Verification items for the finished model (mm, model axes). Face numbers are marked on the shaded views. A direction names the side the tool comes from. Coordinates: 2 decimals unless noted, no trailing zeros. Order: outer loops, then holes, each group sorted by start corner. A loop starts at its lowest first (then second) coordinate and runs counter-clockwise, first axis right, second up. Notation, with made-up numbers: M -37,5 L -11,5 A30 ccw -11,36 Z; hole C -28,-8.5 d7. An arc over 180 degrees is marked long. Write item = value, one per line.
Autodesk Fusion 360 part; units mm, degrees
sketch "Sketch2" plane through (0, 0, 0) normal (1, 0, 0) x (0, 1, 0) in component "Support Batt"
  circle A0 centre (154.2359, 79.3135) radius 4
  line L0 (99.2359, 44.7135) -> (119.2359, 44.7135)
  line L1 (119.2359, 31.7135) -> (119.2359, 44.7135)
  line L2 (99.2359, 31.7135) -> (99.2359, 44.7135)
  line L3 (160.5859, 85.8135) -> (106.4359, 85.8135)
  line L4 (50.5431, 31.7135) -> (52.3447, 31.7135)
  line L5 (52.3447, 31.7135) -> (217.041, 31.7135) construction
  line L6 (96.4359, 75.8135) -> (96.4359, 31.7135)
  line L7 (96.4359, 31.7135) -> (98.9359, 31.7135)
  line L8 (98.9359, 44.7135) -> (119.5359, 44.7135)
  line L9 (119.5359, 44.7135) -> (119.5359, 31.7135)
  line L10 (98.9359, 44.7135) -> (98.9359, 31.7135)
  line L11 (119.5359, 31.7135) -> (122.0359, 31.7135)
  line L12 (154.2359, 83.3135) -> (160.5859, 83.3135) construction
  line L13 (160.5859, 85.8135) -> (160.5859, 70.8135)
  line L14 (158.0859, 70.8135) -> (160.5859, 70.8135)
  line L15 (158.0859, 78.2283) -> (158.0859, 70.8135)
  line L16 (150.3859, 78.2283) -> (150.3859, 70.8135)
  line L17 (150.3859, 70.8135) -> (147.8859, 70.8135)
  line L18 (150.3859, 70.8135) -> (158.0859, 70.8135) construction
  line L19 (154.2359, 79.3135) -> (154.2359, 70.8135) construction
  line L20 (147.8859, 70.8135) -> (147.8859, 71.8135)
  line L21 (137.8859, 81.8135) -> (110.4359, 81.8135)
  line L22 (122.0359, 31.7135) -> (122.0359, 47.7135)
  line L23 (122.0359, 47.7135) -> (110.4359, 47.7135)
  line L24 (100.4359, 57.7135) -> (100.4359, 71.8135)
  arc A1 (110.4359, 81.8135) -> (100.4359, 71.8135) centre (110.4359, 71.8135) ccw
  arc A2 (147.8859, 71.8135) -> (137.8859, 81.8135) centre (137.8859, 71.8135) ccw
  arc A3 (100.4359, 57.7135) -> (110.4359, 47.7135) centre (110.4359, 57.7135) ccw
  arc A4 (158.0859, 78.2283) -> (150.3859, 78.2283) centre (154.2359, 79.3135) ccw
  arc A5 (106.4359, 85.8135) -> (96.4359, 75.8135) centre (106.4359, 75.8135) ccw
  line L25 (114.8859, 81.8135) -> (117.8859, 81.8135)
  line L26 (117.8859, 81.8135) -> (117.8859, 78.8135)
  line L27 (117.8859, 78.8135) -> (114.8859, 78.8135)
  line L28 (114.8859, 78.8135) -> (114.8859, 81.8135)
  line L29 (160.5859, 85.8135) -> (185.5859, 85.8135)
  line L30 (185.5859, 85.8135) -> (185.5859, 82.8135)
  line L31 (185.5859, 82.8135) -> (160.5859, 82.8135)
  line L32 (160.5859, 82.8135) -> (160.5859, 85.8135)
  line L33 (160.5859, 70.8135) -> (185.5859, 82.8135)
  point P0 (96.4359, 85.8135)
  point P1 (100.4359, 81.8135)
  dimension "d2" = 0.3
  dimension "d3" = 0.3
  dimension "d4" = 2.5
  dimension "d5" = 2.5
  dimension "d6" = 2.5
  dimension "d7" = 2.5
  dimension "d8" = 8
  dimension "d9" = 15
  dimension "d10" = 7.7
  dimension "d11" = 2.5
  dimension "d12" = 4
  dimension "d13" = 4
  dimension "d14" = 3
  dimension "d15" = 10
  dimension "d68" = 10
  dimension "d69" = 3
  dimension "d70" = 3
  dimension "d71" = 30
  dimension "d80" = 25
  dimension "d81" = 3
extrude "Extrude1" add sketch "Sketch2" along normal blind 40 contours A0 L0 L3 L6 L7 L8 L9 L10 L11 L13 L14 L15 L16 L17 L20 L21 L22 L23 L24 A1 A2 A3 A4 A5 L25 L32 | L13 L29 L30 L31 L32 | L21 L25 L26 L27 L28 in component "Support Batt"
sketch "Sketch3" plane through (0, 0, 44.7135) normal (0, 0, -1) x (1, 0, 0) in component "Support Batt"
  line L0 (0, -98.9359) -> (0, -119.5359)
  line L1 (0, -119.5359) -> (40, -119.5359)
  line L2 (40, -119.5359) -> (40, -98.9359)
  line L3 (40, -98.9359) -> (0, -98.9359)
  line L4 (0, -109.2359) -> (40, -109.2359) construction
  circle A0 centre (25, -109.2359) radius 1.6
  circle A1 centre (15, -109.2359) radius 1.6
  line L5 (15, -109.2359) -> (25, -109.2359)
  line L6 (20, -109.2359) -> (20, -98.9359)
  circle A2 centre (35, -109.2359) radius 1.6
  circle A3 centre (5, -109.2359) radius 1.6
  dimension "d18" = 3.2
  dimension "d19" = 3.2
  dimension "d33" = 3.2
  dimension "d34" = 3.2
  dimension "d35" = 10
  dimension "d36" = 10
  dimension "d72" = 10
extrude "Extrude2" cut sketch "Sketch3" against normal blind 17 contours A0 | A1 | A2 | A3 in component "Support Batt"
sketch "Sketch4" plane through (0, 0, 47.7135) normal (0, 0, 1) x (-1, 0, 0) in component "Support Batt"
  arc A0 (-26.0583, -110.4359) -> (-23.9417, -110.4359) centre (-25, -109.2359) ccw
  line L0 (-26.0583, -110.4359) -> (-33.9417, -110.4359)
  line L1 (-40, -110.4359) -> (-40, -122.0359)
  line L2 (-40, -122.0359) -> (0, -122.0359)
  line L3 (0, -122.0359) -> (0, -110.4359)
  line L4 (0, -110.4359) -> (-3.9417, -110.4359)
  arc A1 (-16.0583, -110.4359) -> (-13.9417, -110.4359) centre (-15, -109.2359) ccw
  line L5 (-16.0583, -110.4359) -> (-23.9417, -110.4359)
  circle A2 centre (-15, -109.2359) radius 3.25
  circle A3 centre (-25, -109.2359) radius 3.25
  arc A4 (-36.0583, -110.4359) -> (-33.9417, -110.4359) centre (-35, -109.2359) ccw
  line L6 (-36.0583, -110.4359) -> (-40, -110.4359)
  arc A5 (-6.0583, -110.4359) -> (-3.9417, -110.4359) centre (-5, -109.2359) ccw
  line L7 (-6.0583, -110.4359) -> (-13.9417, -110.4359)
  circle A6 centre (-5, -109.2359) radius 3.25
  circle A7 centre (-35, -109.2359) radius 3.25
  dimension "d22" = 6.5
  dimension "d23" = 6.5
  dimension "d37" = 6.5
  dimension "d38" = 6.5
extrude "Extrude3" cut sketch "Sketch4" along normal blind 1.0447 contours A0 L0 L5 A3 | L0 A4 L6 A7 | A1 L5 A2 L7 | L4 A5 L7 A6 picked at (-25.046, -108.9536) picked at (-35.046, -108.9536) picked at (-15.046, -108.9536) picked at (-5.046, -108.9536) in component "Support Batt"
extrude "Extrude3'" add sketch "Sketch2" along normal blind 4 contours L13 L31 L33 in component "Support Batt"
sketch "Sketch5" plane through (40, 0, 0) normal (1, 0, 0) x (0, 1, 0) in component "Support Batt"
  line L0 (158.0859, 70.8135) -> (160.5859, 70.8135)
  line L1 (160.5859, 70.8135) -> (160.5859, 82.8135)
  line L2 (160.5859, 82.8135) -> (185.5859, 82.8135)
  line L3 (185.5859, 82.8135) -> (185.5859, 85.8135)
  line L4 (185.5859, 85.8135) -> (106.4359, 85.8135)
  arc A0 (106.4359, 85.8135) -> (96.4359, 75.8135) centre (106.4359, 75.8135) ccw
  line L5 (96.4359, 75.8135) -> (96.4359, 31.7135)
  line L6 (96.4359, 31.7135) -> (98.9359, 31.7135)
  line L7 (98.9359, 31.7135) -> (98.9359, 44.7135)
  line L8 (98.9359, 44.7135) -> (119.5359, 44.7135)
  line L9 (119.5359, 44.7135) -> (119.5359, 31.7135)
  line L10 (119.5359, 31.7135) -> (122.0359, 31.7135)
  line L11 (122.0359, 31.7135) -> (122.0359, 47.7135)
  line L12 (122.0359, 47.7135) -> (110.4359, 47.7135)
  arc A1 (100.4359, 57.7135) -> (110.4359, 47.7135) centre (110.4359, 57.7135) ccw
  line L13 (100.4359, 57.7135) -> (100.4359, 71.8135)
  arc A2 (110.4359, 81.8135) -> (100.4359, 71.8135) centre (110.4359, 71.8135) ccw
  line L14 (110.4359, 81.8135) -> (114.8859, 81.8135)
  line L15 (114.8859, 81.8135) -> (114.8859, 78.8135)
  line L16 (114.8859, 78.8135) -> (117.8859, 78.8135)
  line L17 (117.8859, 78.8135) -> (117.8859, 81.8135)
  line L18 (117.8859, 81.8135) -> (137.8859, 81.8135)
  arc A3 (147.8859, 71.8135) -> (137.8859, 81.8135) centre (137.8859, 71.8135) ccw
  line L19 (147.8859, 71.8135) -> (147.8859, 70.8135)
  line L20 (147.8859, 70.8135) -> (150.3859, 70.8135)
  line L21
  arc A4 (158.0859, 78.2283) -> (150.3859, 78.2283) centre (154.2359, 79.3135) ccw
  line L22 (158.0859, 78.2283) -> (158.0859, 70.8135)
  line L23 (160.5859, 70.8135) -> (185.5859, 82.8135)
extrude "Extrude4" add sketch "Sketch5" against normal blind 4 in component "Support Batt"
sketch "Sketch4 (1)" plane through (0, 0, 81.8135) normal (0, 0, -1) x (1, 0, 0) in component "Support Batt"
  line L0 (0, -117.8859) -> (0, -137.8859)
  line L1 (0, -137.8859) -> (40, -137.8859)
  line L2 (40, -137.8859) -> (40, -117.8859)
  line L3 (40, -117.8859) -> (0, -117.8859)
  line L4 (0, -147.8859) -> (40, -147.8859)
  line L5 (40, -147.8859) -> (0, -117.8859) construction
  line L6 (0, -158.0859) -> (0, -160.5859) construction
  line L7 (0, -160.5859) -> (4, -160.5859) construction
  line L8 (4, -160.5859) -> (36, -160.5859) construction
  line L9 (36, -160.5859) -> (40, -160.5859) construction
  line L10 (40, -160.5859) -> (40, -158.0859) construction
  line L11 (40, -158.0859) -> (0, -158.0859) construction
  line L12 (0, -160.5859) -> (0, -185.5859) construction
  line L13 (0, -185.5859) -> (4, -185.5859) construction
  line L14 (4, -185.5859) -> (4, -160.5859) construction
  line L15 (4, -160.5859) -> (0, -160.5859) construction
  circle A0 centre (20, -172.0859) radius 10.5
  circle A1 centre (20, -132.8859) radius 11
  line L16 (1.5, -147.8859) -> (38.5, -147.8859)
  line L17 (38.5, -147.8859) -> (38.5, -117.8859)
  line L18 (38.5, -117.8859) -> (1.5, -117.8859)
  line L19 (1.5, -117.8859) -> (1.5, -147.8859)
  line L20 (1.5, -147.8859) -> (38.5, -117.8859) construction
  line L21 (38.5, -147.8859) -> (1.5, -117.8859) construction
  line L22 (20, -158.0859) -> (20, -172.0859)
  point P0 (20, -132.8859)
  dimension "d88" = 21
  dimension "d89" = 22
  dimension "d90" = 37
  dimension "d91" = 30
  dimension "d96" = 14
extrude "Extrude5" cut sketch "Sketch4 (1)" against normal blind 11 contours L1 A1 | L1 A1 | A0 in component "Support Batt"
extrude "Extrude6" cut sketch "Sketch4 (1)" along normal blind 17 contours L1 L4 A1 L16 L17 L19 | L1 A1 picked at (22.1414, -140.7456) in component "Support Batt"
component "Support Batt" placed x (1, 0, 0) y (0, 1, 0) z (0, 0, 1) at (0, 0, 0)
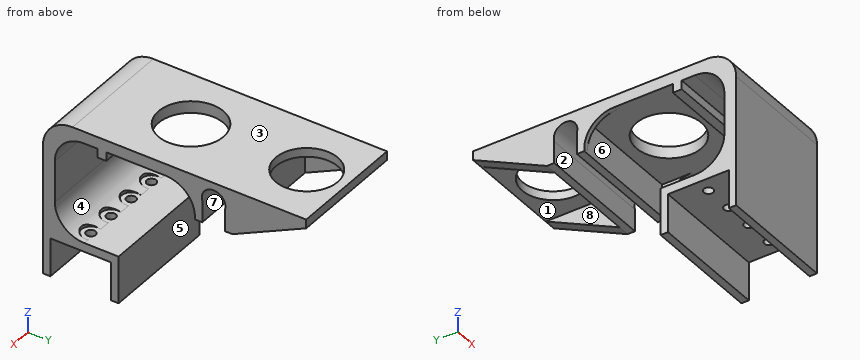
Item 1: Sectioned sample at A-A, the plane z = 39. Enter the section's corners in (x, y).
Report:
outline = M 0,96.44 L 40,96.44 L 40,98.94 L 0,98.94 Z; M 0,119.54 L 40,119.54 L 40,122.04 L 0,122.04 Z
Item 2: Release check for a two-part mould opening along Z. For the marked faces 1, 2, 3 and 4 record: pulls with the +Z half, pulls with the -Z half, needs draft (parallel to the pull), parting line crosses it, or undercut.
Report:
face_1 = pulls with the -Z half
face_2 = needs draft
face_3 = pulls with the +Z half
face_4 = undercut
Item 3: Scan lines: L1, parallel to Y at x = 30, z = 36.5; L2, parallel to Y at x = 25, z = 47; L3, parallel to Z at x = 34.5, y = 111. Record each from-to range of solid material in increasing order. Write a range as from..to.
Report:
L1 = 96.44..98.94, 119.54..122.04
L2 = 96.44..107.64, 110.84..122.04
L3 = 44.71..47.71, 81.81..85.81
Item 4: Sectioned sample at B-B, the plane y = 112. Enter the section's corners in (x, z).
Report:
outline = M 0,44.71 L 40,44.71 L 40,47.71 L 0,47.71 Z; M 0,81.81 L 40,81.81 L 40,85.81 L 0,85.81 Z
Item 5: Tool access check on the marked faces 5, 6, 7 and 8. Record the directions out of +Z, -Z, +X, -X, +Y, -Y that give a thin tool (end or side, any length) a straight path to the whole face; none if there is none.
Report:
face_5 = -Z, +X, -X, +Y
face_6 = -Z
face_7 = -Z, +X, -X
face_8 = -Z, +Y
Item 6: Sectioned sample at D-D, the plane x = 25. Give the number of separate pieces and of enclosed holes in the cut face, then the cut area to 3 significant figures.
Report:
separate_pieces = 4
enclosed_holes = 0
area = 544 mm^2
Item 7: Gauge pin test, flat ends, axial feed: pin 1 (3.5 mm diameter, centred on x = 5, y = 109.24, fed in from -Z); pin 2 (3.5 mm diameter, centred on x = 27, z = 77, fed in from +Y); pin 3 (6 mm diameter, centred on y = 176.5, z = 78, fed in from +X); pin 4 (1.2 mm diameter, centred on x = 12.5, y = 159, fed in from -Z). Record the tip position at first contact, or that the pin passes through.
Report:
pin_1 = 44.71
pin_2 = 160.59
pin_3 = 40
pin_4 = 70.81
